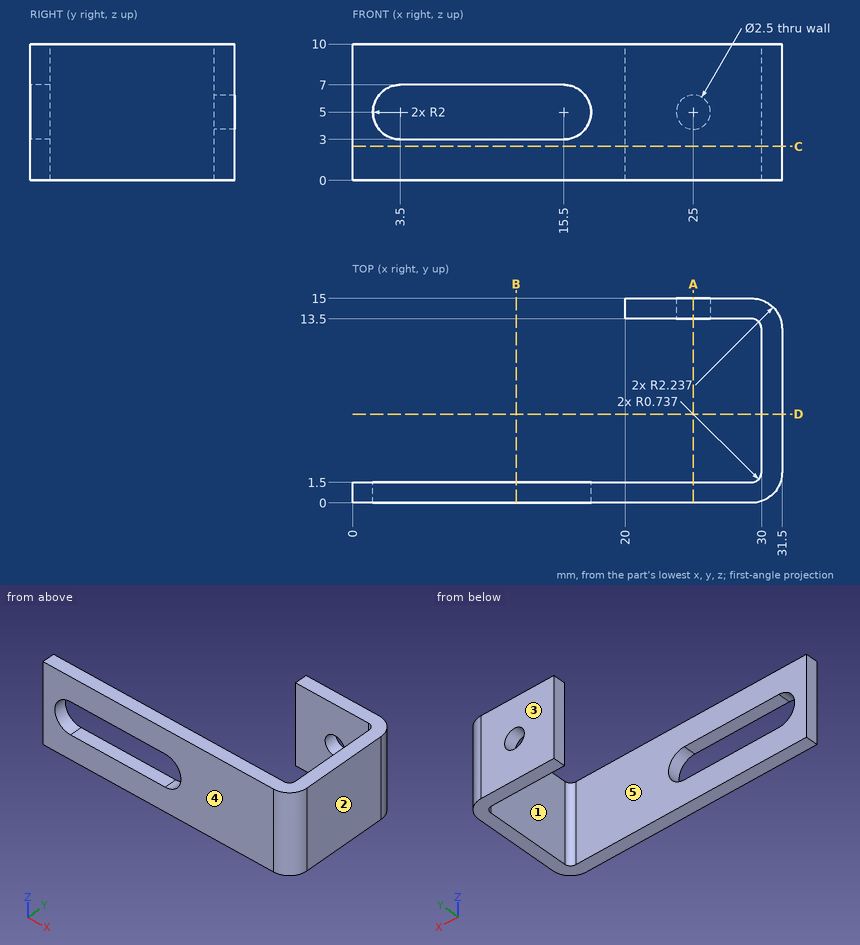
Input: dimensioned drawing with shaded views. Units: mm. Origin: part minimum x, y, z. A direction names the side the tool comes from. Coordinates: 2 decimals unless noted, no trailing zeros. Order: outer loops, then holes, each group sorted by start corner. A loop starts at its lowest first (then second) coordinate and runs counter-clockwise, first axis right, second up.
1. Cut plane C-C, the plane z = 2.5. Return loops of the section in (x, y).
Checked values:
outline: (0, 0) - (29.26, 0) arc R2.24 ccw to (31.5, 2.24) - (31.5, 12.76) arc R2.24 ccw to (29.26, 15) - (20, 15) - (20, 13.5) - (29.26, 13.5) arc R0.74 cw to (30, 12.76) - (30, 2.24) arc R0.74 cw to (29.26, 1.5) - (0, 1.5) - close
2. Contact query for flat-ended pins moving along their axis: P1, Ø1.5, axis at y = 11.5, z = 3, coming from the -X side; P2, Ø1.2, axis at y = 14, z = 2.5, coming from the -X side. Output: stop coordinate, or through.
Checked values:
P1: stops at x = 30
P2: stops at x = 20
3. Cut plane A-A, the plane x = 25. Return loops of the section in (y, z).
Checked values:
outline: (0, 0) - (1.5, 0) - (1.5, 10) - (0, 10) - close; (13.5, 0) - (15, 0) - (15, 3.75) - (13.5, 3.75) - close; (13.5, 6.25) - (15, 6.25) - (15, 10) - (13.5, 10) - close
4. Access query for the marked faces 1 and 2. Directions: +Z, -Z, +X, -X, +Y, -Y. A direction counts if a zero-diameter tool reaches every point of the face in a straight line with its end or side. Return the directions, or none.
Checked values:
face 1: +Z, -Z, -X
face 2: +Z, -Z, +X, +Y, -Y
5. Ray query, line 1 along Z through (x, y) = (25, 14.2); line 2 along Y through (x, z) = (24, 6.5); line 3 along Z through (x, y) = (5, 1.25). Return the intervals inside material, ascending.
Checked values:
line 1: z = 0 to 3.75, 6.25 to 10
line 2: y = 0 to 1.5, 13.5 to 15
line 3: z = 0 to 3, 7 to 10
6. Cut plane B-B, the plane x = 12. Return loops of the section in (y, z).
Checked values:
outline: (0, 0) - (1.5, 0) - (1.5, 3) - (0, 3) - close; (0, 7) - (1.5, 7) - (1.5, 10) - (0, 10) - close
7. Draft query along Y for the marked faces 3, 4 and 5. Return one class per face: +Y half, -Y half, draft (parallel to the pull), parting line (faces both ways), or undercut.
Checked values:
face 3: +Y half
face 4: -Y half
face 5: undercut
8. Cut plane D-D, the plane y = 6.5. Return loops of the section in (x, z), plus the area to 3 significant figures.
Checked values:
outline: (30, 0) - (31.5, 0) - (31.5, 10) - (30, 10) - close
area: 15.0 mm2
